Geometry: see drawing. Coordinates: mm, zero at the bounding-box minimum. A direction names the side the tool comes from. Round coordinates to 2 decimals unless told otherwise and drop trailing zeros. Loops run counter-clockwise (first coordinate to the right, second up) from the corner with the lowest first, then second, coordinate; pieces in that order, holes last. Notation, with made-up numbers: (77.25, -29) - (105.25, -29) arc R31 cw to (105.25, 9) - close; hole circle Ø3 at (19.5, 34.5). An arc over 180 degrees is marked (long way). Write item = value, one per line. Start each with the question number.
Item 1: Access query for the marked faces 1 and 2. Directions: +Z, -Z, +X, -X, +Y, -Y. A direction counts if a zero-diameter tool reaches every point of the face in a straight line with its end or side. Return the directions, or none.
Item 2: Section B-B (z = 26). Return loops of the section in (x, y).
Item 3: Section D-D (x = 12.5). Return loops of the section in (y, z), plus the area to 4 significant figures.
Item 4: Section A-A (x = 52.5). Return loops of the section in (y, z).
Item 5: First-contact query: pin 1 (9 mm diameter, centred on x = 52.5, z = 6, fed in from -Y); pin 2 (1.2 mm diameter, centred on y = 9.5, z = 10, fed in from +X); pin 3 (1.2 mm diameter, centred on y = 9.5, z = 22, fed in from -X). Flat tips, straight axial feed; report the tip coordinate or a pass-through.
Item 6: Section C-C (y = 5.5). Return loops of the section in (x, z).
Item 7: Line query: line 1 (X direction, y = 9.3, z = 6); line 2 (Y direction, x = 69.5, z = 35.8); line 3 (Z direction, x = 9, y = 2.25). Output: solid intervals per line, ascending. Write a range as from..to.
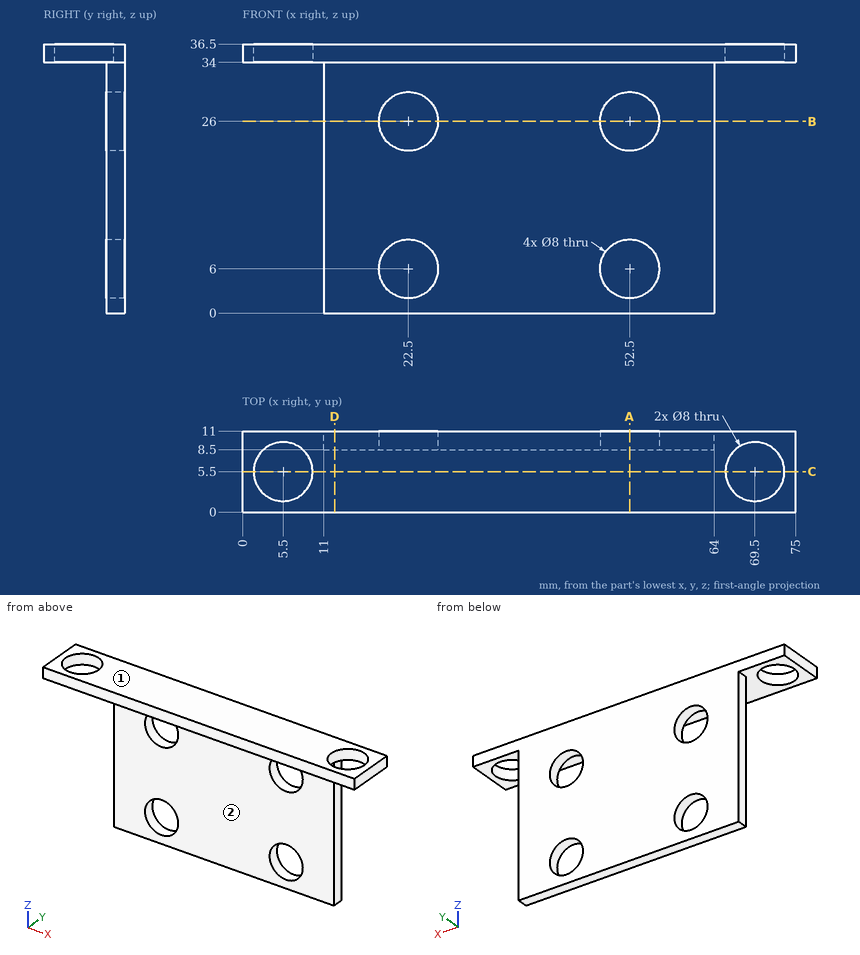
Taken from the geometry:
q1.face_1 = +Z, +X, -X, +Y, -Y
q1.face_2 = -Z, +X, -X, -Y
q2.outline = (11, 8.5) - (18.5, 8.5) - (18.5, 11) - (11, 11) - close; (26.5, 8.5) - (48.5, 8.5) - (48.5, 11) - (26.5, 11) - close; (56.5, 8.5) - (64, 8.5) - (64, 11) - (56.5, 11) - close
q3.outline = (0, 34) - (8.5, 34) - (8.5, 0) - (11, 0) - (11, 36.5) - (0, 36.5) - close
q3.area = 112.5 mm^2
q4.outline = (0, 34) - (8.5, 34) - (8.5, 30) - (11, 30) - (11, 36.5) - (0, 36.5) - close; (8.5, 0) - (11, 0) - (11, 2) - (8.5, 2) - close; (8.5, 10) - (11, 10) - (11, 22) - (8.5, 22) - close
q5.pin_1 = 8.5
q5.pin_2 = 64
q5.pin_3 = 11
q6.outline = (0, 34) - (1.5, 34) - (1.5, 36.5) - (0, 36.5) - close; (9.5, 34) - (65.5, 34) - (65.5, 36.5) - (9.5, 36.5) - close; (73.5, 34) - (75, 34) - (75, 36.5) - (73.5, 36.5) - close
q7.line_1 = 11..18.5, 26.5..48.5, 56.5..64
q7.line_2 = 0..1.5, 9.5..11
q7.line_3 = 34..36.5
